Check sheet for the modelled part. Datum: model origin and axes. Units: mm. A direction names the side the tool comes from. Coordinates: 2 decimals unless noted, no trailing zeros. Order: outer loops, then holes, each group sorted by start corner. A loop starts at its lowest first (then second) coordinate and runs counter-clockwise, first axis right, second up.
1. Gauge pin test, flat ends, axial feed: pin 1 Ø1.5 at (y, z) = (17.5, 32.5) entering from +X; pin 2 Ø2 at (x, y) = (-48, 19) entering from -Z; pin 3 Ø3.5 at (x, y) = (-50.13, 29.09) entering from -Z; pin 4 Ø12 at (x, z) = (-40.5, 10.5) entering from +Y. Record the tip position at first contact, or that the pin passes through.
2. Draft check along X on faces 4 (the cylindrical face through (-68.418, -6.582, 19.72)), 5 (the flat face through (-100, -5, 20)), 6 (the flat face through (-49, -4, 0)). Enter one of: released by +X, released by -X, zero draft, split by the parting line, or undercut.
3. Cross-section at D-D (y = 6). Enter the section's corners in (x, z), then the cut area to 3 significant figures.
4. Cross-section at B-B (x = -50). Enter the section's corners in (y, z), then the cut area to 3 significant figures.
5. Cross-section at A-A (z = 11.5). Enter the section's corners in (x, y).
6. Cross-section at C-C (z = 36). Enter the section's corners in (x, y).
7. Thickness scan on line 1 (Y direction, x = -24.5, z = 26.5); line 2 (Z direction, x = -37, y = 11); line 3 (Y direction, x = -37, z = 19.5). Record the ranges inside material, lowest first.
8. Set-up check for faces 1 (the cylindrical face through (-31.505, -6.656, 19.72)), 2 (the cylindrical face through (-69, 13, 38)), 3 (the flat face through (-30, 12, 33)): record each of +Z, -Z, +X, -X, +Y, -Y from which the full face is reachable in a straight line by a thin tool's end or side.
```python
from build123d import *

# Parameters (mm, degrees)
F0_W          = 100
F0_H          = 40
F1_DEPTH      = 10
F3_DEPTH      = 10
F4_W          = 40
F4_H          = 3
F5_DEPTH      = 174
F6_W          = 40
F6_H          = 4.7629310191
F7_DEPTH      = 40.001
F8_R          = 2.85
F9_DEPTH      = 40.001
F10_T1_DEPTH  = 40
F10_T3_DEPTH  = 40
F10_T5_DEPTH  = 35
F10_T7_DEPTH  = 35
F10_T9_DEPTH  = 35
F10_T11_DEPTH = 35
F10_T13_DEPTH = 25
F10_T16_ANGLE = 180


# Not quite as in the source:
# - a fillet or chamfer that OpenCascade refuses, or shapes differently, is made with other operations: its cross-section is extruded or revolved along the edge and cut away or added
# - two fillets or chamfers of one size are made in one step
# - an extrude ends at something that could not be found from the text; its depth is read off the source's solid


with BuildPart() as f1:
    # F0 (on Front) → F1 (new body)
    with BuildSketch(Plane.XZ):
        with Locations((-50, 20)):
            Rectangle(F0_W, F0_H)
    extrude(amount=F1_DEPTH)

    # F2 (on face) → F3 (join)
    with BuildSketch(Plane.XY.offset(40)):
        with BuildLine():
            Line((-70, 25), (-70, 0))
            Line((-70, 0), (-70, -10))
            Line((-70, -10), (-30, -10))
            Line((-30, -10), (-30, 0))
            Line((-30, 0), (-30, 25))
            ThreePointArc((-30, 25), (-50, 45), (-70, 25))
        make_face()
        with BuildLine():
            Line((-70, 25), (-70, 0))
            Line((-70, 0), (-30, 0))
            Line((-30, 0), (-30, 25))
            ThreePointArc((-30, 25), (-50, 45), (-70, 25))
        make_face()
    extrude(amount=-F3_DEPTH)

    # F4 (on face) → F5 (cut, through all)
    with BuildSketch(Plane.XY.offset(40)):
        with Locations((-50, -8.5)):
            Rectangle(F4_W, F4_H)
    extrude(amount=F5_DEPTH, mode=Mode.SUBTRACT)

    # F6 (on face) → F7 (cut, through all)
    with BuildSketch(Plane.XY.offset(40)):
        with Locations((-50, -7.6185344905)):
            Rectangle(F6_W, F6_H)
    extrude(amount=-F7_DEPTH, mode=Mode.SUBTRACT)

    # F8 (on face) → F9 (cut, through all)
    with BuildSketch(Plane.XY.offset(40)):
        with Locations((-50.1293092966, 29.0948301554)):
            Circle(F8_R)
    extrude(amount=-F9_DEPTH, mode=Mode.SUBTRACT)

    # F10: fillet of radius 5 on 9 edges, made by hand

    # F10_s2 → F10_t1 (join)
    with BuildSketch(Plane.XY):
        with BuildLine():
            ThreePointArc((-30, -10), (-31.543677094, -6.6186891705), (-34.9943766676, -5.2370689809))
            Line((-34.9943766676, -5.2370689809), (-30, -5.2370689809))
            Line((-30, -5.2370689809), (-30, -10))
        make_face()
    extrude(amount=F10_T1_DEPTH)

    # F10_s4 → F10_t3 (join)
    with BuildSketch(Plane.XY):
        with BuildLine():
            ThreePointArc((-65.0056233324, -5.2370689809), (-68.456322906, -6.6186891705), (-70, -10))
            Line((-70, -10), (-70, -5.2370689809))
            Line((-70, -5.2370689809), (-65.0056233324, -5.2370689809))
        make_face()
    extrude(amount=F10_T3_DEPTH)

    # F10_s6 → F10_t5 (cut)
    with BuildSketch(Plane.XZ.offset(-12.5)):
        with BuildLine():
            ThreePointArc((-5, 0), (-1.4644660941, 1.4644660941), (0, 5))
            Line((0, 5), (0, 0))
            Line((0, 0), (-5, 0))
        make_face()
    extrude(amount=F10_T5_DEPTH, mode=Mode.SUBTRACT)

    # F10_s8 → F10_t7 (cut)
    with BuildSketch(Plane.XZ.offset(-12.5)):
        with BuildLine():
            ThreePointArc((-95, 0), (-98.5355339059, 1.4644660941), (-100, 5))
            Line((-100, 5), (-100, 0))
            Line((-100, 0), (-95, 0))
        make_face()
    extrude(amount=F10_T7_DEPTH, mode=Mode.SUBTRACT)

    # F10_s10 → F10_t9 (cut)
    with BuildSketch(Plane.XZ.offset(-12.5)):
        with BuildLine():
            ThreePointArc((-5, 40), (-1.4644660941, 38.5355339059), (0, 35))
            Line((0, 35), (0, 40))
            Line((0, 40), (-5, 40))
        make_face()
    extrude(amount=F10_T9_DEPTH, mode=Mode.SUBTRACT)

    # F10_s12 → F10_t11 (cut)
    with BuildSketch(Plane.XZ.offset(-12.5)):
        with BuildLine():
            ThreePointArc((-95, 40), (-98.5355339059, 38.5355339059), (-100, 35))
            Line((-100, 35), (-100, 40))
            Line((-100, 40), (-95, 40))
        make_face()
    extrude(amount=F10_T11_DEPTH, mode=Mode.SUBTRACT)

    # F10_s14 → F10_t13 (cut)
    with BuildSketch(Plane.XZ.offset(-25)):
        with BuildLine():
            ThreePointArc((-70, 35), (-68.5355339059, 38.5355339059), (-65, 40))
            Line((-65, 40), (-70, 40))
            Line((-70, 40), (-70, 35))
        make_face()
        with BuildLine():
            ThreePointArc((-30, 35), (-31.4644660941, 38.5355339059), (-35, 40))
            Line((-35, 40), (-30, 40))
            Line((-30, 40), (-30, 35))
        make_face()
    extrude(amount=F10_T13_DEPTH, mode=Mode.SUBTRACT)

    # F10_s15 → F10_t16 (revolve, cut)
    with BuildSketch(Plane.XZ.offset(-25)):
        with BuildLine():
            ThreePointArc((-35, 40), (-31.4644660941, 38.5355339059), (-30, 35))
            Line((-30, 35), (-30, 40))
            Line((-30, 40), (-35, 40))
        make_face()
    revolve(axis=Axis((-50, 25, 40), (0, 0, 1)), revolution_arc=F10_T16_ANGLE, mode=Mode.SUBTRACT)


solid = f1.part
```
Data:
1. pin 1: stops at x = -30
1. pin 2: stops at z = 30
1. pin 3: passes through
1. pin 4: stops at y = 0
2. face 4: undercut
2. face 5: released by -X
2. face 6: zero draft
3. outline: (-70, 30) - (-30, 30) - (-30, 35) arc R5 ccw to (-35, 40) - (-65, 40) arc R5 ccw to (-70, 35) - close
3. area: 389 mm2
4. outline: (-5.24, 0) - (0, 0) - (0, 30) - (26.25, 30) - (26.25, 40) - (-5.24, 40) - close; (31.94, 30) - (45, 30) - (45, 35) arc R5 ccw to (40, 40) - (31.94, 40) - close
4. area: 597 mm2
5. outline: (-100, -10) - (-70, -10) arc R5 cw to (-65.01, -5.24) - (-34.99, -5.24) arc R5 cw to (-30, -10) - (0, -10) - (0, 0) - (-100, 0) - close
6. outline: (-99.9, -10) - (-70, -10) arc R5 cw to (-65.01, -5.24) - (-34.99, -5.24) arc R5 cw to (-30, -10) - (-0.1, -10) - (-0.1, 0) - (-30.1, 0) - (-30.1, 25) arc R19.9 ccw to (-69.9, 25) - (-69.9, 0) - (-99.9, 0) - close; hole circle Ø5.7 at (-50.13, 29.09)
7. line 1: y = -10 to 0
7. line 2: z = 30 to 40
7. line 3: y = -5.24 to 0
8. face 1: +Z, -Z, -Y
8. face 2: +Z, -X, +Y
8. face 3: +Z, -Z, +X, +Y
